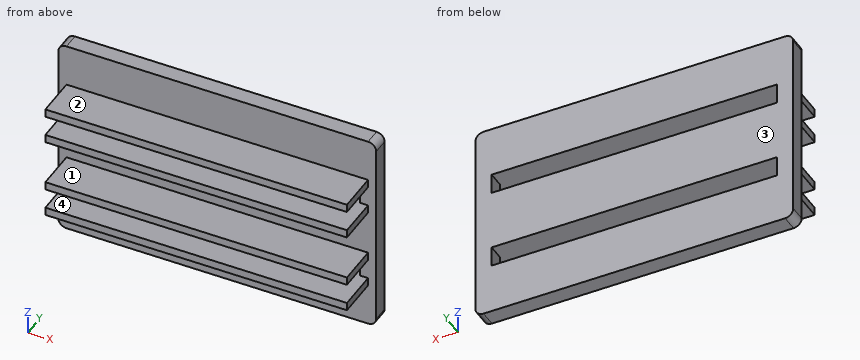
```python
from build123d import *

# Parameters (mm, degrees)
BOSS_EXTRUDE1_DEPTH = 5.08
SKETCH4_W           = 88.9
SKETCH4_H           = 6.35
CUT_EXTRUDE2_DEPTH  = 5.08
SKETCH6_W           = 2.54
SKETCH6_H           = 12.7
BOSS_EXTRUDE2_DEPTH = 46.99


with BuildPart() as part:
    # Sketch2 → Boss-Extrude1 (new body)
    with BuildSketch(Plane(origin=(0, 0, 0), x_dir=(1, 0, 0), z_dir=(0, 1, 0))):
        with BuildLine():
            Line((-46.99, 31.75), (46.99, 31.75))
            ThreePointArc((46.99, 31.75), (48.786051224, 31.006051224), (49.53, 29.21))
            Line((49.53, 29.21), (49.53, -29.21))
            ThreePointArc((49.53, -29.21), (48.786051224, -31.006051224), (46.99, -31.75))
            Line((46.99, -31.75), (-46.99, -31.75))
            ThreePointArc((-46.99, -31.75), (-48.786051224, -31.006051224), (-49.53, -29.21))
            Line((-49.53, -29.21), (-49.53, 29.21))
            ThreePointArc((-49.53, 29.21), (-48.786051224, 31.006051224), (-46.99, 31.75))
        make_face()
    extrude(amount=BOSS_EXTRUDE1_DEPTH)

    # Sketch4 → Cut-Extrude2 (cut)
    with BuildSketch(Plane(origin=(0, 0, 0), x_dir=(1, 0, 0), z_dir=(0, 1, 0))):
        with Locations((0, 12.7)):
            Rectangle(SKETCH4_W, SKETCH4_H)
        with Locations((0, -12.7)):
            Rectangle(SKETCH4_W, SKETCH4_H)
    extrude(amount=CUT_EXTRUDE2_DEPTH, mode=Mode.SUBTRACT)

    # Sketch6 → Boss-Extrude2 (add, symmetric)
    with BuildSketch(Plane(origin=(0, 0, 0), x_dir=(0, 0, -1), z_dir=(1, 0, 0))):
        with Locations((-17.145, -6.35)):
            Rectangle(SKETCH6_W, SKETCH6_H)
        with Locations((-8.255, -6.35)):
            Rectangle(SKETCH6_W, SKETCH6_H)
        with Locations((8.255, -6.35)):
            Rectangle(SKETCH6_W, SKETCH6_H)
        with Locations((17.145, -6.35)):
            Rectangle(SKETCH6_W, SKETCH6_H)
    extrude(amount=BOSS_EXTRUDE2_DEPTH, both=True)


solid = part.part
```
Can you work these out from the model? Positions are in its coordinate system, mm. Face numbers are marked on the shaded views. A direction names the side the tool comes from. Coordinates: 2 decimals unless noted, no trailing zeros. Loops run counter-clockwise (first coordinate to the right, second up) from the corner with the lowest first, then second, coordinate; pieces in that order, holes last. Notation, with made-up numbers: (89.25, 31) -> (123.25, 31) arc R18 cw to (123.25, 52) -> close; hole circle Ø4 at (79.5, 34). An arc over 180 degrees is marked (long way). Answer as a JSON object with one key per item and string values.
1) Imagine slicing it at A-A (z = -14.5). Please give me the cut outline in (x, y).
Results:
{"outline": "(-49.53, 0) -> (-44.45, 0) -> (-44.45, 5.08) -> (-49.53, 5.08) -> close; (44.45, 0) -> (49.53, 0) -> (49.53, 5.08) -> (44.45, 5.08) -> close"}
2) For P1, Ø3, axis at y = -5.5, z = -17.5, coming from the -X side; P2, Ø5, axis at x = -33, z = 23, coming from the -Y side; P3, Ø4, axis at x = 28.5, y = -5, coming from the +Z side (3 decimals), each with a flat end and sliding along its axis, tell me the tip position at first contact or that it passes through.
Results:
{"P1": "stops at x = -46.99", "P2": "stops at y = 0", "P3": "stops at z = 18.415"}
3) Imagine slicing it at D-D (y = 2.75). Please give me the cut outline in (x, z) (3 decimals).
Results:
{"outline": "(-49.53, -29.21) arc R2.54 ccw to (-46.99, -31.75) -> (46.99, -31.75) arc R2.54 ccw to (49.53, -29.21) -> (49.53, 29.21) arc R2.54 ccw to (46.99, 31.75) -> (-46.99, 31.75) arc R2.54 ccw to (-49.53, 29.21) -> close; hole (-44.45, -15.875) -> (44.45, -15.875) -> (44.45, -9.525) -> (-44.45, -9.525) -> close; hole (-44.45, 9.525) -> (44.45, 9.525) -> (44.45, 15.875) -> (-44.45, 15.875) -> close"}
4) Thinking about a two-plate mould opening in X: for the marked faces 3 and 4, which applies, pulls with the +X half, pulls with the -X half, needs draft (parallel to the pull), parting line crosses it, or undercut?
Results:
{"face 3": "needs draft", "face 4": "undercut"}
5) Imagine slicing it at B-B (y = -9.25). Please give me the cut outline in (x, z) (3 decimals).
Results:
{"outline": "(-46.99, -18.415) -> (46.99, -18.415) -> (46.99, -15.875) -> (-46.99, -15.875) -> close; (-46.99, -9.525) -> (46.99, -9.525) -> (46.99, -6.985) -> (-46.99, -6.985) -> close; (-46.99, 6.985) -> (46.99, 6.985) -> (46.99, 9.525) -> (-46.99, 9.525) -> close; (-46.99, 15.875) -> (46.99, 15.875) -> (46.99, 18.415) -> (-46.99, 18.415) -> close"}
6) If I drill on line 1 (Z direction, x = 25, y = -6.5) (3 decimals); line 2 (Z direction, x = 31, y = 1.25) (3 decimals); line 3 (Y direction, x = 45, z = -15), over which ranges is the centre line in solid material (lowest first)?
Results:
{"line 1": "z = -18.415 to -15.875, -9.525 to -6.985, 6.985 to 9.525, 15.875 to 18.415", "line 2": "z = -31.75 to -15.875, -9.525 to 9.525, 15.875 to 31.75", "line 3": "y = 0 to 5.08"}
7) For the marked faces 1 and 2, which set-ups out of +Z, -Z, +X, -X, +Y, -Y let a thin tool reach every point of the face, with its end or its side?
Results:
{"face 1": "+X, -X, -Y", "face 2": "+Z, +X, -X, -Y"}
8) Imagine slicing it at C-C (x = -35.5). Please give me the cut outline in (y, z) (3 decimals), then the cut area to 3 significant figures.
Results:
{"outline": "(-12.7, -18.415) -> (0, -18.415) -> (0, -31.75) -> (5.08, -31.75) -> (5.08, -15.875) -> (-12.7, -15.875) -> close; (-12.7, -9.525) -> (5.08, -9.525) -> (5.08, 9.525) -> (-12.7, 9.525) -> (-12.7, 6.985) -> (0, 6.985) -> (0, -6.985) -> (-12.7, -6.985) -> close; (-12.7, 15.875) -> (5.08, 15.875) -> (5.08, 31.75) -> (0, 31.75) -> (0, 18.415) -> (-12.7, 18.415) -> close", "area": "387 mm^2"}
